```python
from build123d import *

# Parameters (mm, degrees)
BOSS_EXTRUDE1_DEPTH = 12.7


with BuildPart() as part:
    # Sketch1 → Boss-Extrude1 (new body)
    with BuildSketch(Plane.XY):
        with BuildLine():
            Line((-20.574, -61.084457743), (578.569437198, -61.084457743))
            ThreePointArc((578.569437198, -61.084457743), (581.981934524, -59.670955069), (583.395437198, -56.258457743))
            Line((583.395437198, -56.258457743), (583.395437198, -36.911371471))
            add(Edge.make_bspline(
                [(583.395437198, -36.911371471), (610.890329995, -46.033932746), (618.425396158, -69.67439137), (618.425396158, -96.114416703)],
                knots=[0, 0, 0, 0, 1, 1, 1, 1], degree=3))
            Line((618.425396158, -96.114416703), (618.425396158, -572.727698858))
            add(Edge.make_bspline(
                [(583.395437198, -631.93074409), (610.890329995, -622.808182814), (618.425396158, -599.167724191), (618.425396158, -572.727698858)],
                knots=[0, 0, 0, 0, 1, 1, 1, 1], degree=3))
            Line((583.395437198, -631.93074409), (583.395437198, -612.583657817))
            ThreePointArc((583.395437198, -612.583657817), (581.981934524, -609.171160491), (578.569437198, -607.757657817))
            Line((578.569437198, -607.757657817), (-20.574, -607.757657817))
            ThreePointArc((-20.574, -607.757657817), (-23.986497326, -609.171160491), (-25.4, -612.583657817))
            Line((-25.4, -612.583657817), (-25.4, -631.93074409))
            add(Edge.make_bspline(
                [(-25.4, -631.93074409), (-52.894892797, -622.808182814), (-60.42995896, -599.167724191), (-60.42995896, -572.727698858)],
                knots=[0, 0, 0, 0, 1, 1, 1, 1], degree=3))
            Line((-60.42995896, -572.727698858), (-60.42995896, -96.114416703))
            add(Edge.make_bspline(
                [(-25.4, -36.911371471), (-52.894892797, -46.033932746), (-60.42995896, -69.67439137), (-60.42995896, -96.114416703)],
                knots=[0, 0, 0, 0, 1, 1, 1, 1], degree=3))
            Line((-25.4, -36.911371471), (-25.4, -56.258457743))
            ThreePointArc((-25.4, -56.258457743), (-23.986497326, -59.670955069), (-20.574, -61.084457743))
        make_face()
    extrude(amount=BOSS_EXTRUDE1_DEPTH)


solid = part.part
```
For this review, take the finished solid that the model builds, in its own axes (mm). Round coordinates to 2 decimals unless told otherwise and drop trailing zeros. Order: outer loops, then holes, each group sorted by start corner. A loop starts at its lowest first (then second) coordinate and runs counter-clockwise, first axis right, second up.
Q1. Wall thickness on line 1 (Y direction, x = 285, z = 1.75); line 2 (X direction, y = -607, z = 9.5); line 3 (Y direction, x = -23, z = 3): over which ranges is each line inside the solid? List them lowest first.
Findings below:
line 1: y = -607.76 to -61.08
line 2: x = -54.12 to 612.11
line 3: y = -608.41 to -60.43
Q2. We need section A-A, the plane x = 462.5. Give the boundary of the cut face in (y, z).
Findings below:
outline: (-607.76, 0) - (-61.08, 0) - (-61.08, 12.7) - (-607.76, 12.7) - close
Q3. Insertion check: P1, Ø5, axis at x = 181, z = 7.5, coming from the -Y side; P2, Ø4, axis at y = -623, z = 6, coming from the -X side; P3, Ø4, axis at y = -618.5, z = 7.5, coming from the +X side. Each pin has a flat end and moves straight along its axis. Give the tip position at first contact, or say it passes through.
Findings below:
P1: stops at y = -607.76
P2: stops at x = -44.19
P3: stops at x = 606.3
